Autodesk Inventor part; units mm, degrees
ref_plane "YZ Plane" through (0, 0, 0) normal (1, 0, 0) x (0, 1, 0)
ref_plane "XZ Plane" through (0, 0, 0) normal (0, 1, 0) x (-1, 0, 0)
ref_plane "XY Plane" through (0, 0, 0) normal (0, 0, 1) x (1, 0, 0)
sketch "Sketch8" plane through (0, 0, 0) normal (0, 0, 1) x (1, 0, 0)
  line L0 (0, 2897) -> (1200, 2897)
  line L1 (1200, 2897) -> (1200, 0)
  line L2 (1200, 0) -> (0, 0)
  line L3 (0, 0) -> (0, 2897)
  line L4 (0, 2897) -> (1200, 0) construction
  line L5 (1200, 2897) -> (0, 0) construction
  line L6 (947, 0) -> (1097, 150)
  line L7 (1097, 150) -> (1147, 2897)
  line L8 (0, 700) -> (1200, 700)
  line L9 (1112.5806, 1006) -> (837.057, 700)
  line L10 (110.253, 0) -> (110.253, 700)
  point P0 (600, 1448.5)
  point P1 (1107.0109, 700)
  dimension "d43" = 1200
  dimension "d44" = 2897
  dimension "d45" = 53
  dimension "d46" = 947
  dimension "d47" = 150
  dimension "d48" = 103
  dimension "d49" = 700
  dimension "d55" = 306
  dimension "d57" = 110.253
  dimension "d61" = 48
extrude "Plate4" add sketch "Sketch8" against normal blind 3 contours L7 L8 L9 | L8 L7 L6 L2 L10
chamfer "Corner Chamfer1" distance 6 angle 45 2 edges at (947, 0, -1.5) (1097, 150, -1.5)
chamfer "Corner Chamfer2" distance 6 angle 45 1 edges at (1112.5806, 1006, -1.5)
equation "\"d50\" = Thickness"
equation "\"BendReliefWidth\" = Thickness"
equation "\"BendReliefDepth\" = 0.5 * Thickness"
equation "\"CornerReliefSize\" = 4 * Thickness"
equation "\"MinimumRemnant\" = 2 * Thickness"
equation "\"TransitionRadius\" = BendRadius"
equation "\"JacobiRadiusSize\" = BendRadius"
equation "\"GapSize\" = Thickness"
properties part number "BSH 015 board cone 5" material "09g2s"
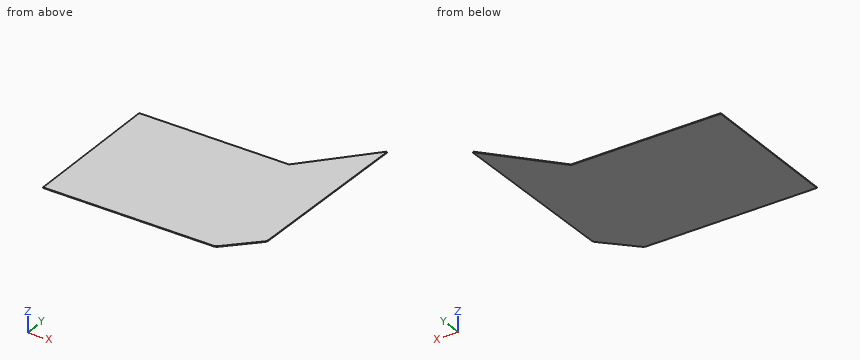
Work out the finished part from the listing and answer in its coordinate system (mm). Coordinates: 2 decimals unless noted, no trailing zeros. Write each loop counter-clockwise with the first axis right and the second up, starting at its lowest first coordinate (ties: lowest second). Pieces come first, ordered by that corner, then holes. Notation, with made-up numbers: M 88,-32.5 L 130,-32.5 A15 ccw 130,-7.5 Z; hole C 42.5,77.25 d11. An arc over 180 degrees is marked long. Write item = value, one per line.
1. The part is cut by section C-C (y = 65). Determine the outline of the cut face in (x, z), then the cut area to 3 significant figures.
Solution:
outline = M 110.25,-3 L 1012,-3 L 1012,0 L 110.25,0 Z
area = 2,710 mm2
2. Flat-ended cylindrical pins translate along their axes: pin 1 (5 mm diameter, centred on x = 681.5, y = 632, fed in from +Z); pin 2 (0.9 mm diameter, centred on x = 340, z = -1, fed in from +Y). Find the tip coordinate at first contact, or state that the pin passes through.
Solution:
pin_1 = 0
pin_2 = 700
3. The part is cut by section A-A (z = -1.65). Determine the outline of the cut face in (x, y), then the cut area to 3 significant figures.
Solution:
outline = M 110.25,0 L 941,0 L 951.24,4.24 L 1092.76,145.76 L 1097.11,156 L 1112.47,1000 L 1108.57,1001.54 L 837.06,700 L 110.25,700 Z
area = 723,000 mm2
4. Straight lines are drawn through the part: line 1 (Y direction, x = 682, z = -1.3); line 2 (X direction, y = 315, z = -2.35); line 3 (X direction, y = 256.5, z = -0.2). For each, find the intervals that lie inside material, in ascending order. Write a range as from..to.
Solution:
line_1 = 0..700
line_2 = 110.25..1100
line_3 = 110.25..1098.94
5. The part is cut by section B-B (x = 540.5). Determine the outline of the cut face in (y, z), then the cut area to 3 significant figures.
Solution:
outline = M 0,-3 L 700,-3 L 700,0 L 0,0 Z
area = 2,100 mm2
